Design review of the part built by this model. Coordinates are the model's own, in mm. A direction names the side the tool comes from. Give positions to 0.01 mm unless a question says otherwise; leave off trailing zeros. Order: outer loops, then holes, each group sorted by start corner. A loop starts at its lowest first (then second) coordinate and runs counter-clockwise, first axis right, second up. Notation, with made-up numbers: M 58.5,34 L 111.5,34 A18 ccw 111.5,54 Z; hole C 79.5,65.25 d10. An arc over 180 degrees is marked long. Answer as a JSON object with one key per item and string values.
from build123d import *

# Parameters (mm, degrees)
SKETCH1_R           = 48.25
BOSS_EXTRUDE1_DEPTH = 5
SKETCH2_W           = 17.162038191
SKETCH2_H           = 56.822210482
SKETCH2_W_2         = 16.152506533
SKETCH2_H_2         = 65.186901365
CUT_EXTRUDE1_DEPTH  = 8
SKETCH3_R           = 30
CUT_EXTRUDE2_DEPTH  = 8
SKETCH4_R           = 1.75
CUT_EXTRUDE3_DEPTH  = 10
SKETCH6_R           = 1.75
CUT_EXTRUDE4_DEPTH  = 10
CIRPATTERN2_COUNT   = 2
CIRPATTERN2_ANGLE   = 45
CIRPATTERN3_COUNT   = 2
CIRPATTERN3_ANGLE   = 45
SKETCH7_R           = 1.75
CUT_EXTRUDE5_DEPTH  = 10
CIRPATTERN4_COUNT   = 2
CIRPATTERN4_ANGLE   = 45
CIRPATTERN5_COUNT   = 2
CIRPATTERN5_ANGLE   = 315
SKETCH8_R           = 54
BOSS_EXTRUDE3_DEPTH = 33.7
SKETCH10_R          = 3
CUT_EXTRUDE6_DEPTH  = 3.5
SKETCH12_R          = 3
CUT_EXTRUDE7_DEPTH  = 3.5
SKETCH11_R          = 3
CUT_EXTRUDE8_DEPTH  = 3.5
BOSS_EXTRUDE4_DEPTH = 34
SKETCH14_R          = 2
CUT_EXTRUDE9_DEPTH  = 34


with BuildPart() as part:
    # Sketch1 → Boss-Extrude1 (new body)
    with BuildSketch(Plane.XY):
        Circle(SKETCH1_R)
    extrude(amount=-BOSS_EXTRUDE1_DEPTH)

    # Sketch2 → Cut-Extrude1 (cut)
    with BuildSketch(Plane.XY):
        with Locations((-54.831019095, 0)):
            Rectangle(SKETCH2_W, SKETCH2_H)
        with Locations((54.326253267, -4.182345442)):
            Rectangle(SKETCH2_W_2, SKETCH2_H_2)
    extrude(amount=-CUT_EXTRUDE1_DEPTH, mode=Mode.SUBTRACT)

    # Sketch3 → Cut-Extrude2 (cut)
    with BuildSketch(Plane.XY):
        Circle(SKETCH3_R)
    extrude(amount=-CUT_EXTRUDE2_DEPTH, mode=Mode.SUBTRACT)

    # Sketch4 → Cut-Extrude3 (cut)
    with BuildSketch(Plane.XY):
        with Locations((-42.5, 0)):
            Circle(SKETCH4_R)
        with Locations((42.5, 0)):
            Circle(SKETCH4_R)
    extrude(amount=-CUT_EXTRUDE3_DEPTH, mode=Mode.SUBTRACT)

    # Sketch6 → Cut-Extrude4 (cut)
    with BuildSketch(Plane.XY):
        with Locations((0, 44.5)):
            Circle(SKETCH6_R)
    cut_extrude4 = extrude(amount=-CUT_EXTRUDE4_DEPTH, mode=Mode.SUBTRACT)

    # CirPattern2: Cut-Extrude4 ×2 about axis
    cirpattern2_axis = Axis((0, 0, -8), (0, 0, 1))
    for i in range(1, CIRPATTERN2_COUNT):
        add(cut_extrude4.rotate(cirpattern2_axis, i * CIRPATTERN2_ANGLE / (CIRPATTERN2_COUNT - 1)), mode=Mode.SUBTRACT)

    # CirPattern3: Cut-Extrude4 ×2 about axis
    cirpattern3_axis = Axis((0, 0, -8), (0, 0, -1))
    for i in range(1, CIRPATTERN3_COUNT):
        add(cut_extrude4.rotate(cirpattern3_axis, i * CIRPATTERN3_ANGLE / (CIRPATTERN3_COUNT - 1)), mode=Mode.SUBTRACT)

    # Sketch7 → Cut-Extrude5 (cut)
    with BuildSketch(Plane.XY):
        with Locations((0, -44.5)):
            Circle(SKETCH7_R)
    cut_extrude5 = extrude(amount=-CUT_EXTRUDE5_DEPTH, mode=Mode.SUBTRACT)

    # CirPattern4: Cut-Extrude5 ×2 about axis
    cirpattern4_axis = Axis((0, 0, -8), (0, 0, 1))
    for i in range(1, CIRPATTERN4_COUNT):
        add(cut_extrude5.rotate(cirpattern4_axis, i * CIRPATTERN4_ANGLE / (CIRPATTERN4_COUNT - 1)), mode=Mode.SUBTRACT)

    # CirPattern5: Cut-Extrude5 ×2 about axis
    cirpattern5_axis = Axis((0, 0, -8), (0, 0, 1))
    for i in range(1, CIRPATTERN5_COUNT):
        add(cut_extrude5.rotate(cirpattern5_axis, i * CIRPATTERN5_ANGLE / (CIRPATTERN5_COUNT - 1)), mode=Mode.SUBTRACT)

    # Sketch10 → Cut-Extrude6 (cut)
    with BuildSketch(Plane(origin=(0, 0, -5), x_dir=(-1, 0, 0), z_dir=(0, 0, -1))):
        with Locations((-31.466251763, 31.466251763)):
            Circle(SKETCH10_R)
    extrude(amount=-CUT_EXTRUDE6_DEPTH, mode=Mode.SUBTRACT)

    # Sketch12 → Cut-Extrude7 (cut)
    with BuildSketch(Plane(origin=(0, 0, -5), x_dir=(-1, 0, 0), z_dir=(0, 0, -1))):
        with Locations((-42.5, 0)):
            Circle(SKETCH12_R)
    extrude(amount=-CUT_EXTRUDE7_DEPTH, mode=Mode.SUBTRACT)

    # Sketch11 → Cut-Extrude8 (cut)
    with BuildSketch(Plane(origin=(0, 0, -5), x_dir=(-1, 0, 0), z_dir=(0, 0, -1))):
        with Locations((31.466251763, -31.466251763)):
            Circle(SKETCH11_R)
    extrude(amount=-CUT_EXTRUDE8_DEPTH, mode=Mode.SUBTRACT)


with BuildPart() as body_2:
    # Sketch8 → Boss-Extrude3 (new body)
    with BuildSketch(Plane(origin=(0, 0, -5), x_dir=(-1, 0, 0), z_dir=(0, 0, -1))):
        Circle(SKETCH8_R)
        with BuildLine():
            Line((-46.25, 13.747727085), (-46.25, -13.747727085))
            ThreePointArc((-46.25, -13.747727085), (0, -48.25), (46.25, -13.747727085))
            Line((46.25, -13.747727085), (46.25, 13.747727085))
            ThreePointArc((46.25, 13.747727085), (0, 48.25), (-46.25, 13.747727085))
        make_face(mode=Mode.SUBTRACT)
    extrude(amount=-BOSS_EXTRUDE3_DEPTH)


    add(part.part)  # Boss-Extrude4 merges part
    # Sketch13 → Boss-Extrude4 (add)
    with BuildSketch(Plane(origin=(0, 0, -5), x_dir=(-1, 0, 0), z_dir=(0, 0, -1))):
        with BuildLine():
            Line((-54, 0), (-54, -62.045472978))
            Line((-54, -62.045472978), (54, -62.045472978))
            Line((54, -62.045472978), (54, 0))
            ThreePointArc((54, 0), (0, -54), (-54, 0))
        make_face()
    extrude(amount=-BOSS_EXTRUDE4_DEPTH)

    # Sketch14 → Cut-Extrude9 (cut)
    with BuildSketch(Plane(origin=(0, 0, -5), x_dir=(-1, 0, 0), z_dir=(0, 0, -1))):
        with Locations((-24, -53.783750327)):
            Circle(SKETCH14_R)
        with Locations((24, -53.783750327)):
            Circle(SKETCH14_R)
    extrude(amount=-CUT_EXTRUDE9_DEPTH, mode=Mode.SUBTRACT)


solid = body_2.part
(1) We need section C-C (x = -24). Write out the cut boundary in (y, z).
Checked values:
{"outline": "M -62.05,-5 L -55.78,-5 L -55.78,29 L -62.05,29 Z; M -51.78,-5 L -18,-5 L -18,0 L -41.86,0 L -41.86,28.7 L -48.37,28.7 L -48.37,29 L -51.78,29 Z; M 18,-5 L 48.37,-5 L 48.37,28.7 L 41.86,28.7 L 41.86,0 L 18,0 Z"}
(2) We need section A-A (y = -44.5). Write out the cut boundary in (x, z), plus the area to 3 significant figures.
Checked values:
{"outline": "M -54,-5 L -1.75,-5 L -1.75,0 L -18.65,0 L -18.65,28.7 L -30.59,28.7 L -30.59,29 L -54,29 Z; M 1.75,-5 L 54,-5 L 54,29 L 30.59,29 L 30.59,28.7 L 18.65,28.7 L 18.65,0 L 1.75,0 Z", "area": "2,570 mm^2"}
(3) We need section B-B (x = 42.5). Write out the cut boundary in (y, z).
Checked values:
{"outline": "M -62.05,-5 L -3,-5 L -3,-1.5 L -1.75,-1.5 L -1.75,0 L -22.84,0 L -22.84,28.7 L -33.31,28.7 L -33.31,29 L -62.05,29 Z; M 1.75,-1.5 L 3,-1.5 L 3,-5 L 33.31,-5 L 33.31,28.7 L 22.84,28.7 L 22.84,0 L 1.75,0 Z"}
(4) Draft analysis for pull direction X (two halves, no side actions). For faces 5 (the flat face through (-11, -29, -5)), 6 (the flat face through (54, -31, 12)), 7 (the cylindrical face through (33.847, 29.641, -3.274)), state which applies: +X half, -X half, draft (parallel to the pull), parting line (faces both ways), or undercut.
Checked values:
{"face 5": "draft", "face 6": "+X half", "face 7": "undercut"}
(5) Insertion check: pin 1 (5 mm diameter, centred on x = 30.5, y = 32.5, fed in from -Z); pin 2 (9.5 mm diameter, centred on x = 42.5, y = 0, fed in from +Z); pin 3 (5 mm diameter, centred on x = 29.5, y = -23, fed in from +Z); pin 4 (4 mm diameter, centred on x = 13, z = 22, fed in from +Y). Each pin has a flat end and moves straight along its axis. Give the tip position at first contact, or say it passes through.
Checked values:
{"pin 1": "stops at z = -5", "pin 2": "stops at z = 28.7", "pin 3": "stops at z = 0", "pin 4": "stops at y = 52.87"}
(6) Tool access review of faces 1 (the flat face through (-33, -33, -1.5)), 2 (the flat face through (8, -48, 28.7)), 3 (the cylindrical face through (-0.866, 48.242, 14.149)), 4 (the flat face through (1, -62.045, 12)): name each direction out of +Z, -Z, +X, -X, +Y, -Y from which nothing blocks a thin tool from reaching the whole face with its end or side.
Checked values:
{"face 1": "-Z", "face 2": "+Z, +Y", "face 3": "+Z", "face 4": "+Z, -Z, +X, -X, -Y"}
(7) To check wall thickness, follow L1, parallel to X at y = -1, z = 1.5; L2, parallel to Y at x = -17, z = 17; L3, parallel to Z at x = 27, y = 20. State the ranges of each line that lie inside material, in increasing order. Write a range as from..to.
Checked values:
{"L1": "x = -54..-46.25, 46.25..54", "L2": "y = -62.05..-45.16, 45.16..51.25", "L3": "z = -5..0"}
(8) We need section D-D (z = 16.5). Write out the cut boundary in (x, y), plus the area to 3 significant figures.
Checked values:
{"outline": "M -54,-62.05 L 54,-62.05 L 54,0 A54 ccw -54,0 Z; hole M -46.25,-13.75 A48.25 ccw 46.25,-13.75 L 46.25,13.75 A48.25 ccw -46.25,13.75 Z; hole C -24,-53.78 d4; hole C 24,-53.78 d4", "area": "4,020 mm^2"}
